Build history of the part. All positions in model axes, mm. A direction names the side the tool comes from. Give positions to 0.01 mm unless a question says otherwise; leave off trailing zeros. Order: outer loops, then holes, each group sorted by start corner. A loop starts at its lowest first (then second) coordinate and runs counter-clockwise, first axis right, second up. Notation, with made-up numbers: M 10.5,59.25 L 36.5,59.25 A26 cw 36.5,74.25 Z; hole C -25.5,-27 d11. An arc over 180 degrees is marked long. One line per item, written item: value.
from build123d import *

# Parameters (mm, degrees)
SKETCH1_R           = 10
BOSS_EXTRUDE1_DEPTH = 30
SKETCH2_W           = 90
SKETCH2_H           = 70
BOSS_EXTRUDE2_DEPTH = 10


with BuildPart() as part:
    # Sketch1 → Boss-Extrude1 (new body)
    with BuildSketch(Plane.XY):
        with BuildLine():
            Line((0, 35), (20, 35))
            Line((20, 35), (20, -35))
            Line((20, -35), (0, -35))
            ThreePointArc((0, -35), (-35, 0), (0, 35))
        make_face()
        with Locations((-17.5, 0)):
            Circle(SKETCH1_R, mode=Mode.SUBTRACT)
    extrude(amount=BOSS_EXTRUDE1_DEPTH)

    # Sketch2 → Boss-Extrude2 (add)
    with BuildSketch(Plane(origin=(20, 0, 0), x_dir=(0, 0, -1), z_dir=(1, 0, 0))):
        with Locations((-15, 0)):
            Rectangle(SKETCH2_W, SKETCH2_H)
    extrude(amount=BOSS_EXTRUDE2_DEPTH)


solid = part.part
1) Tool access for faces 4 (the face through (18, -35, 16)), 5 (the face through (20, 0, -15)), 6 (the face through (-1, 0, 30)): list every direction of +Z, -Z, +X, -X, +Y, -Y with a clear straight run to the whole face (end or side of a thin tool).
Check values:
face 4: +Z, -Z, +X, -X, -Y
face 5: -Z, -X, +Y, -Y
face 6: +Z, -X, +Y, -Y
2) Saw through at C-C, the plane z = -24. Write the cut outline in (x, y).
Check values:
outline: M 20,-35 L 30,-35 L 30,35 L 20,35 Z
3) Drill centre lines: probe 1 along X at (y, z) = (12.5, -16.5); probe 2 along Z at (x, y) = (8.5, 6); probe 3 along Y at (x, z) = (-17, 21). Where is each one in solid material? Low to high. Write a range as from..to.
Check values:
probe 1: 20..30
probe 2: 0..30
probe 3: -30.59..-9.99, 9.99..30.59
4) Pin check, flat tips, straight feed: pin 1 (10 mm diameter, centred on y = 7, z = 49, fed in from -X); pin 2 (12 mm diameter, centred on x = -6, y = 22, fed in from -Z); pin 3 (4 mm diameter, centred on x = -5.5, z = 6.5, fed in from +Y). Stop position of each tip, or through.
Check values:
pin 1: x = 20
pin 2: z = 0
pin 3: y = 34.82
5) Saw through at D-D, the plane y = -27. Write the cut outline in (x, z).
Check values:
outline: M -22.27,0 L 20,0 L 20,-30 L 30,-30 L 30,60 L 20,60 L 20,30 L -22.27,30 Z
6) Mould opens along Y. For faces 1 (the face through (-7.96, 3, 14.79)), 2 (the face through (25, 0, 60)), 3 (the face through (18, 35, 16)) say: released by +Y, released by -Y, zero draft, split by the parting line, or undercut.
Check values:
face 1: undercut
face 2: zero draft
face 3: released by +Y
7) Saw through at B-B, the plane x = -17.5. Write the cut outline in (y, z).
Check values:
outline: M -30.31,0 L -10,0 L -10,30 L -30.31,30 Z; M 10,0 L 30.31,0 L 30.31,30 L 10,30 Z
8) Saw through at A-A, the plane y = 0. Write the cut outline in (x, z), then the cut area to 3 significant figures.
Check values:
outline: M -35,0 L -27.5,0 L -27.5,30 L -35,30 Z; M -7.5,0 L 20,0 L 20,-30 L 30,-30 L 30,60 L 20,60 L 20,30 L -7.5,30 Z
area: 1,950 mm^2
